Read the model definition and answer for the solid it produces. Units are mm, in the model's axes. A direction names the side the tool comes from. Give positions to 0.01 mm unless a question says otherwise; leave off trailing zeros. Order: outer loops, then holes, each group sorted by start corner. A loop starts at its lowest first (then second) coordinate and runs counter-clockwise, first axis right, second up.
```python
from build123d import *

# Parameters (mm, degrees)
BOSS_EXTRUDE1_DEPTH = 3
SKETCH2_W           = 130
SKETCH2_H           = 1.5
BOSS_EXTRUDE2_DEPTH = 3
SKETCH3_W           = 1.5
SKETCH3_H           = 18.75
BOSS_EXTRUDE3_DEPTH = 3
SKETCH4_R           = 2
CUT_EXTRUDE1_DEPTH  = 97.213304693


with BuildPart() as part:
    # Sketch1 → Boss-Extrude1 (new body)
    with BuildSketch(Plane(origin=(0, 0, 0), x_dir=(1, 0, 0), z_dir=(0, 1, 0))):
        Polygon((65, 38.88), (68, 38.88), (68, 12.76), (65, 12.76), (65, -13.06), (68, -13.06), (68, -39.18), (65, -39.18), (65, -65), (39.18, -65), (39.18, -68), (13.06, -68), (13.06, -65), (-12.76, -65), (-12.76, -68), (-38.88, -68), (-38.88, -65), (-64.7, -65), (-68, -65), (-68, -38.88), (-65, -38.88), (-65, -13.06), (-68, -13.06), (-68, 13.06), (-65, 13.06), (-65, 38.88), (-68, 38.88), (-68, 65), (-65, 65), (-65, 68), (-38.88, 68), (-38.88, 65), (-13.06, 65), (-13.06, 68), (13.06, 68), (13.06, 65), (38.88, 65), (38.88, 68), (65, 68), (65, 64.7), align=None)
        with BuildLine():
            Line((22.627762262, -60), (-22.627762262, -60))
            ThreePointArc((-22.627762262, -60), (-45.343222344, -45.343222344), (-60, -22.627762262))
            Line((-60, -22.627762262), (-60, 22.627762262))
            ThreePointArc((-60, 22.627762262), (-45.343222344, 45.343222344), (-22.627762262, 60))
            Line((-22.627762262, 60), (22.627762262, 60))
            ThreePointArc((22.627762262, 60), (45.343222344, 45.343222344), (60, 22.627762262))
            Line((60, 22.627762262), (60, -22.627762262))
            ThreePointArc((60, -22.627762262), (45.343222344, -45.343222344), (22.627762262, -60))
        make_face(mode=Mode.SUBTRACT)
    extrude(amount=BOSS_EXTRUDE1_DEPTH)

    # Sketch2 → Boss-Extrude2 (add, through all)
    with BuildSketch(Plane(origin=(0, 3, 0), x_dir=(1, 0, 0), z_dir=(0, 1, 0))):
        with Locations((0, 60.75)):
            Rectangle(SKETCH2_W, SKETCH2_H)
        with Locations((0, 40.5)):
            Rectangle(SKETCH2_W, SKETCH2_H)
        with Locations((0, 20.25)):
            Rectangle(SKETCH2_W, SKETCH2_H)
        Rectangle(SKETCH2_W, SKETCH2_H)
        with Locations((0, -20.25)):
            Rectangle(SKETCH2_W, SKETCH2_H)
        with Locations((0, -40.5)):
            Rectangle(SKETCH2_W, SKETCH2_H)
        with Locations((0, -60.75)):
            Rectangle(SKETCH2_W, SKETCH2_H)
    extrude(amount=-BOSS_EXTRUDE2_DEPTH)

    # Sketch3 → Boss-Extrude3 (add, through all)
    with BuildSketch(Plane(origin=(0, 3, 0), x_dir=(1, 0, 0), z_dir=(0, 1, 0))):
        with Locations((-30.375, -30.375)):
            Rectangle(SKETCH3_W, SKETCH3_H)
        with Locations((-30.375, -10.125)):
            Rectangle(SKETCH3_W, SKETCH3_H)
        with BuildLine():
            Line((-29.625, -41.25), (-31.125, -41.25))
            Line((-31.125, -41.25), (-31.125, -56.064694773))
            ThreePointArc((-31.125, -56.064694773), (-30.377679063, -56.473110768), (-29.625, -56.87156583))
            Line((-29.625, -56.87156583), (-29.625, -41.25))
        make_face()
        with Locations((0, -30.375)):
            Rectangle(SKETCH3_W, SKETCH3_H)
        with Locations((-30.375, 30.375)):
            Rectangle(SKETCH3_W, SKETCH3_H)
        with Locations((-30.375, 10.125)):
            Rectangle(SKETCH3_W, SKETCH3_H)
        with Locations((0, -10.125)):
            Rectangle(SKETCH3_W, SKETCH3_H)
        with Locations((0, -50.625)):
            Rectangle(SKETCH3_W, SKETCH3_H)
        with BuildLine():
            Line((-31.125, 56.064694773), (-31.125, 41.25))
            Line((-31.125, 41.25), (-29.625, 41.25))
            Line((-29.625, 41.25), (-29.625, 56.87156583))
            ThreePointArc((-29.625, 56.87156583), (-30.377679063, 56.473110768), (-31.125, 56.064694773))
        make_face()
        with Locations((30.375, -30.375)):
            Rectangle(SKETCH3_W, SKETCH3_H)
        with Locations((0, 30.375)):
            Rectangle(SKETCH3_W, SKETCH3_H)
        with Locations((0, 10.125)):
            Rectangle(SKETCH3_W, SKETCH3_H)
        with Locations((30.375, -10.125)):
            Rectangle(SKETCH3_W, SKETCH3_H)
        with BuildLine():
            Line((31.125, -41.25), (29.625, -41.25))
            Line((29.625, -41.25), (29.625, -56.87156583))
            ThreePointArc((29.625, -56.87156583), (30.377679063, -56.473110768), (31.125, -56.064694773))
            Line((31.125, -56.064694773), (31.125, -41.25))
        make_face()
        with Locations((0, 50.625)):
            Rectangle(SKETCH3_W, SKETCH3_H)
        with Locations((30.375, 30.375)):
            Rectangle(SKETCH3_W, SKETCH3_H)
        with Locations((30.375, 10.125)):
            Rectangle(SKETCH3_W, SKETCH3_H)
        with BuildLine():
            Line((29.625, 56.87156583), (29.625, 41.25))
            Line((29.625, 41.25), (31.125, 41.25))
            Line((31.125, 41.25), (31.125, 56.064694773))
            ThreePointArc((31.125, 56.064694773), (30.377679063, 56.473110768), (29.625, 56.87156583))
        make_face()
    extrude(amount=-BOSS_EXTRUDE3_DEPTH)

    # Sketch4 → Cut-Extrude1 (cut, through all)
    with BuildSketch(Plane(origin=(0, 3, 0), x_dir=(1, 0, 0), z_dir=(0, 1, 0))):
        with Locations(Location((-52.5, 52.5, 0), (0, 0, 270))):
            Circle(SKETCH4_R)
        with Locations(Location((52.5, 52.5, 0), (0, 0, 270))):
            Circle(SKETCH4_R)
        with Locations(Location((52.5, -52.5, 0), (0, 0, 270))):
            Circle(SKETCH4_R)
        with Locations(Location((-52.5, -52.5, 0), (0, 0, 270))):
            Circle(SKETCH4_R)
    extrude(amount=-CUT_EXTRUDE1_DEPTH, mode=Mode.SUBTRACT)


solid = part.part
```
1) For a pull along X with two mould halves and no side action, classify faces 1 (the face through (-52, 1, -68)), 2 (the face through (-41, 2, 39.75)), 3 (the face through (68, 1, -26)) as released by +X, released by -X, zero draft, split by the parting line, or undercut.
Final values:
face 1: zero draft
face 2: undercut
face 3: released by +X
2) The part is cut by section C-C on z = -52.5. Determine the outline of the cut face in (x, y) (3 decimals), and give its area (3 significant figures).
Final values:
outline: (-68, 0) - (-54.5, 0) - (-54.5, 3) - (-68, 3) - close; (-50.5, 0) - (-36.821, 0) - (-36.821, 3) - (-50.5, 3) - close; (-31.125, 0) - (-29.625, 0) - (-29.625, 3) - (-31.125, 3) - close; (-0.75, 0) - (0.75, 0) - (0.75, 3) - (-0.75, 3) - close; (29.625, 0) - (31.125, 0) - (31.125, 3) - (29.625, 3) - close; (36.821, 0) - (50.5, 0) - (50.5, 3) - (36.821, 3) - close; (54.5, 0) - (65, 0) - (65, 3) - (54.5, 3) - close
area: 168 mm2
3) Given pin 1 (0.8 mm diameter, centred on y = 2, z = 22, fed in from -X); pin 2 (0.9 mm diameter, centred on y = 2, z = -10.5, fed in from +X); pin 3 (1 mm diameter, centred on x = -22, y = 1.5, fed in from -Z), each flat-ended and moving along its own axis, determine where each tip first touches the part or whether it passes through.
Final values:
pin 1: stops at x = -65
pin 2: stops at x = 65
pin 3: stops at z = -65
4) The part is cut by section B-B on x = -11. Determine the outline of the cut face in (y, z), and give its area (3 significant figures).
Final values:
outline: (0, -68) - (3, -68) - (3, -60) - (0, -60) - close; (0, -41.25) - (3, -41.25) - (3, -39.75) - (0, -39.75) - close; (0, -21) - (3, -21) - (3, -19.5) - (0, -19.5) - close; (0, -0.75) - (3, -0.75) - (3, 0.75) - (0, 0.75) - close; (0, 19.5) - (3, 19.5) - (3, 21) - (0, 21) - close; (0, 39.75) - (3, 39.75) - (3, 41.25) - (0, 41.25) - close; (0, 60) - (3, 60) - (3, 65) - (0, 65) - close
area: 61.5 mm2
5) Consider L1, parallel to X at y = 1.85, z = -5 (3 decimals); L2, parallel to X at y = 1.05, z = 17 (3 decimals). Determine where each line is inside the solid, lowest interval first.
Final values:
L1: x = -68 to -60, -31.125 to -29.625, -0.75 to 0.75, 29.625 to 31.125, 60 to 65
L2: x = -65 to -60, -31.125 to -29.625, -0.75 to 0.75, 29.625 to 31.125, 60 to 68
6) The part is cut by section A-A on z = -9. Determine the outline of the cut face in (x, y) (3 decimals), and give its area (3 significant figures).
Final values:
outline: (-68, 0) - (-60, 0) - (-60, 3) - (-68, 3) - close; (-31.125, 0) - (-29.625, 0) - (-29.625, 3) - (-31.125, 3) - close; (-0.75, 0) - (0.75, 0) - (0.75, 3) - (-0.75, 3) - close; (29.625, 0) - (31.125, 0) - (31.125, 3) - (29.625, 3) - close; (60, 0) - (65, 0) - (65, 3) - (60, 3) - close
area: 52.5 mm2
7) The part is cut by section D-D on y = 0.5. Count the separate pieces of the cut face and the enclosed holes in it, and give its area (3 significant figures).
Final values:
separate pieces: 1
enclosed holes: 28
area: 6,540 mm2
8) A tool of negligible diameter and unlimited length cuts with its end or side. For faces 4 (the face through (-26, 1, -65)), 5 (the face through (65, 1, 52)), 6 (the face through (45, 2, 0.75)), 7 (the face through (-26, 1, 68)), from which of +Z, -Z, +X, -X, +Y, -Y can it reach the whole face along a straight path? Write none if from no direction.
Final values:
face 4: -Z, +Y, -Y
face 5: +Z, +X, +Y, -Y
face 6: +Y, -Y
face 7: +Z, +X, -X, +Y, -Y
